```python
from build123d import *

# Parameters (mm, degrees)
SKETCH1_R           = 31.5
SKETCH1_R_2         = 26
BOSS_EXTRUDE1_DEPTH = 35
SKETCH1_9_W         = 20
SKETCH1_9_H         = 6
SKETCH1_9_R         = 12
BOSS_EXTRUDE2_DEPTH = 21
BOSS_EXTRUDE4_START = -21
SKETCH1_13_W        = 20
SKETCH1_13_H        = 6
BOSS_EXTRUDE4_DEPTH = 42
FILLET1_R           = 72
CUT_EXTRUDE1_START  = -2.5
SKETCH1_10_W        = 150
SKETCH1_10_H        = 6
CUT_EXTRUDE1_DEPTH  = 270.112775841
SKETCH1_11_R        = 5
BOSS_EXTRUDE3_DEPTH = 21
SKETCH1_12_R        = 5
CUT_EXTRUDE2_DEPTH  = 14


with BuildPart() as part:
    # Sketch1 → Boss-Extrude1 (new, symmetric)
    with BuildSketch(Plane.XY):
        Circle(SKETCH1_R)
        Circle(SKETCH1_R_2, mode=Mode.SUBTRACT)
    extrude(amount=BOSS_EXTRUDE1_DEPTH, both=True)

    # Sketch1<9> → Boss-Extrude2 (add, symmetric)
    with BuildSketch(Plane.XY):
        with BuildLine():
            ThreePointArc((240.444891614, 14.661169931), (230.786453061, 10.283897205), (220.260411081, 9))
            Line((220.260411081, 9), (90, 13))
            Line((90, 13), (28.692333471, 13))
            ThreePointArc((28.692333471, 13), (31.5, 0), (28.692333471, -13))
            Line((28.692333471, -13), (90, -13))
            Line((90, -13), (220.260411081, -9))
            ThreePointArc((220.260411081, -9), (230.786453061, -10.283897205), (240.444891614, -14.661169931))
            ThreePointArc((240.444891614, -14.661169931), (267.5, 0), (240.444891614, 14.661169931))
        make_face()
        with Locations((80, 0)):
            Rectangle(SKETCH1_9_W, SKETCH1_9_H, mode=Mode.SUBTRACT)
        with Locations(Location((250, 0, 0), (0, 0, 180))):
            Circle(SKETCH1_9_R, mode=Mode.SUBTRACT)
    extrude(amount=BOSS_EXTRUDE2_DEPTH, both=True)

    # Sketch1<13> → Boss-Extrude4 (add)
    with BuildSketch(Plane.XY.offset(BOSS_EXTRUDE4_START)):
        with Locations((80, 0)):
            Rectangle(SKETCH1_13_W, SKETCH1_13_H)
    extrude(amount=BOSS_EXTRUDE4_DEPTH)

    # Fillet1
    fillet1_edges = [part.edges().sort_by_distance(p)[0] for p in [
        (28.692333471, 13, 0),
        (28.692333471, -13, 0),
    ]]
    fillet(fillet1_edges, radius=FILLET1_R)

    # Sketch1<10> → Cut-Extrude1 (cut, through all)
    with BuildSketch(Plane.XY.offset(CUT_EXTRUDE1_START)):
        with Locations((145, 0)):
            Rectangle(SKETCH1_10_W, SKETCH1_10_H)
        with BuildLine():
            ThreePointArc((220, 3), (223, 0), (220, -3))
            Line((220, -3), (220, 3))
        make_face()
        with BuildLine():
            Line((70, -3), (70, 3))
            ThreePointArc((70, 3), (67, 0), (70, -3))
        make_face()
    cut_extrude1 = extrude(amount=-CUT_EXTRUDE1_DEPTH, mode=Mode.SUBTRACT)

    # Mirror1: Cut-Extrude1 across plane
    add(cut_extrude1.mirror(Plane.XY), mode=Mode.SUBTRACT)

    # Sketch1<11> → Boss-Extrude3 (add, symmetric)
    with BuildSketch(Plane.XY):
        with BuildLine():
            Line((28.692333471, 13), (90, 13))
            ThreePointArc((90, 13), (54.465075477, 23.652725045), (28.950381961, 50.582482314))
            ThreePointArc((28.950381961, 50.582482314), (18.050555131, 58.582082925), (4.938808192, 55.283306326))
            ThreePointArc((4.938808192, 55.283306326), (-15.790013542, 43.424058768), (-39.257670087, 38.997446139))
            ThreePointArc((-39.257670087, 38.997446139), (-49.580007549, 33.5540347), (-51.376901133, 22.023529412))
            ThreePointArc((-51.376901133, 22.023529412), (-47.925892025, 0), (-51.376901133, -22.023529412))
            ThreePointArc((-51.376901133, -22.023529412), (-49.563579479, -33.576990734), (-39.201221462, -38.998442596))
            ThreePointArc((-39.201221462, -38.998442596), (-14.290092236, -43.85808942), (7.387013832, -57.059740797))
            ThreePointArc((7.387013832, -57.059740797), (18.504940725, -60.078747549), (27.655633909, -53.079639433))
            ThreePointArc((27.655633909, -53.079639433), (53.274598705, -24.401721259), (90, -13))
            Line((90, -13), (28.692333471, -13))
            ThreePointArc((28.692333471, -13), (-31.5, 0), (28.692333471, 13))
        make_face()
        with Locations(Location((16, -47.322365932, 0), (0, 0, 180))):
            Circle(SKETCH1_11_R, mode=Mode.SUBTRACT)
        with Locations(Location((-39, -26, 0), (0, 0, 180))):
            Circle(SKETCH1_11_R, mode=Mode.SUBTRACT)
        with Locations(Location((-39, 26, 0), (0, 0, 180))):
            Circle(SKETCH1_11_R, mode=Mode.SUBTRACT)
        with Locations(Location((15, 43, 0), (0, 0, 180))):
            Circle(SKETCH1_11_R, mode=Mode.SUBTRACT)
    extrude(amount=BOSS_EXTRUDE3_DEPTH, both=True)

    # Sketch1<12> → Cut-Extrude2 (cut, symmetric)
    with BuildSketch(Plane.XY):
        with BuildLine():
            Line((28.692333471, 13), (90, 13))
            ThreePointArc((90, 13), (54.465075477, 23.652725045), (28.950381961, 50.582482314))
            ThreePointArc((28.950381961, 50.582482314), (18.050555131, 58.582082925), (4.938808192, 55.283306326))
            ThreePointArc((4.938808192, 55.283306326), (-15.790013542, 43.424058768), (-39.257670087, 38.997446139))
            ThreePointArc((-39.257670087, 38.997446139), (-49.580007549, 33.5540347), (-51.376901133, 22.023529412))
            ThreePointArc((-51.376901133, 22.023529412), (-47.925892025, 0), (-51.376901133, -22.023529412))
            ThreePointArc((-51.376901133, -22.023529412), (-49.563579479, -33.576990734), (-39.201221462, -38.998442596))
            ThreePointArc((-39.201221462, -38.998442596), (-14.290092236, -43.85808942), (7.387013832, -57.059740797))
            ThreePointArc((7.387013832, -57.059740797), (18.504940725, -60.078747549), (27.655633909, -53.079639433))
            ThreePointArc((27.655633909, -53.079639433), (53.274598705, -24.401721259), (90, -13))
            Line((90, -13), (28.692333471, -13))
            ThreePointArc((28.692333471, -13), (-31.5, 0), (28.692333471, 13))
        make_face()
        with Locations(Location((16, -47.322365932, 0), (0, 0, 180))):
            Circle(SKETCH1_12_R, mode=Mode.SUBTRACT)
        with Locations(Location((-39, -26, 0), (0, 0, 180))):
            Circle(SKETCH1_12_R, mode=Mode.SUBTRACT)
        with Locations(Location((-39, 26, 0), (0, 0, 180))):
            Circle(SKETCH1_12_R, mode=Mode.SUBTRACT)
        with Locations(Location((15, 43, 0), (0, 0, 180))):
            Circle(SKETCH1_12_R, mode=Mode.SUBTRACT)
    extrude(amount=CUT_EXTRUDE2_DEPTH, both=True, mode=Mode.SUBTRACT)


solid = part.part
```
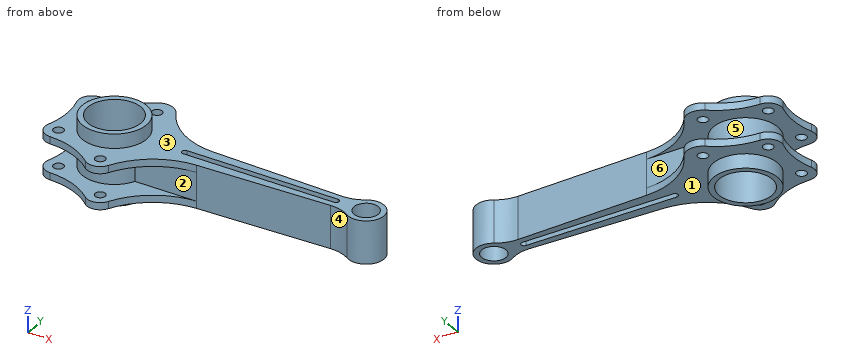
Verification items for the finished model (mm, model axes). Face numbers are marked on the shaded views. A direction names the side the tool comes from. Coordinates: 2 decimals unless noted, no trailing zeros. Order: outer loops, then holes, each group sorted by start corner. A loop starts at its lowest first (then second) coordinate and runs counter-clockwise, first axis right, second up. Notation, with made-up numbers: (64, 15.5) - (103, 15.5) arc R25 ccw to (103, 42.5) - close; hole circle Ø5 at (68.25, 10). An arc over 180 degrees is marked (long way). Return JSON: item names as keys, results as strings.
(1) Thickness scan on line 1 along Y through (x, z) = (-39, -16.25); line 2 along Z through (x, y) = (31, -21); line 3 along Y through (x, z) = (250, 4.5). Record the ranges inside material, lowest first.
Filled sheet:
{"line 1": "y = -39 to -31, -21 to 21, 31 to 39", "line 2": "z = -21 to -14, 14 to 21", "line 3": "y = -17.5 to -12, 12 to 17.5"}
(2) Section check C-C, the plane x = -8. Record the cut outline in (y, z).
Filled sheet:
{"outline": "(-46.65, -21) - (-30.47, -21) - (-30.47, -35) - (-24.74, -35) - (-24.74, 35) - (-30.47, 35) - (-30.47, 21) - (-46.65, 21) - (-46.65, 14) - (-30.47, 14) - (-30.47, -14) - (-46.65, -14) - close; (24.74, -35) - (30.47, -35) - (30.47, -21) - (46.83, -21) - (46.83, -14) - (30.47, -14) - (30.47, 14) - (46.83, 14) - (46.83, 21) - (30.47, 21) - (30.47, 35) - (24.74, 35) - close"}
(3) Access from +Z, -Z, +X, -X, +Y, -Y to the whole of each face (thin tool, end or side, straight path). Record for the marked faces 3, 4, 5 and 6.
Filled sheet:
{"face 3": "+Z", "face 4": "+Z, -Z, -Y", "face 5": "none", "face 6": "+Y"}
(4) Section check B-B, the plane z = -8. Record the cut outline in (x, y), and give its area (3 significant figures).
Filled sheet:
{"outline": "(28.69, -13) - (90, -13) - (220.26, -9) arc R35 cw to (240.44, -14.66) arc R17.5 ccw (long way) to (240.44, 14.66) arc R35 cw to (220.26, 9) - (90, 13) - (28.69, 13) arc R31.5 ccw (long way) to start; hole circle Ø52 at (0, 0); hole (70, -3) - (220, -3) arc R3 ccw to (220, 3) - (70, 3) arc R3 ccw to start; hole circle Ø24 at (250, 0)", "area": "5,250 mm^2"}
(5) Section check D-D, the plane x = 212.5. Record the cut outline in (y, z).
Filled sheet:
{"outline": "(-9.24, -21) - (-3, -21) - (-3, -2.5) - (3, -2.5) - (3, -21) - (9.24, -21) - (9.24, 21) - (3, 21) - (3, 2.5) - (-3, 2.5) - (-3, 21) - (-9.24, 21) - close"}
(6) Mould release check, pull along X, two halves, no side actions. Record for the marked faces 1 and 2: pulls with the +X half, pulls with the -X half, needs draft (parallel to the pull), parting line crosses it, or undercut.
Filled sheet:
{"face 1": "needs draft", "face 2": "undercut"}
(7) Section check A-A, the plane y = 0. Give the number of separate pieces and of enclosed holes in the cut face, and give its area (3 significant figures).
Filled sheet:
{"separate pieces": "3", "enclosed holes": "0", "area": "4,130 mm^2"}
(8) Go/stop test with flat-tipped pins: pin 1 (9 mm diameter, centred on x = 117, z = -9, fed in from -Y); pin 2 (8 mm diameter, centred on x = 207.5, y = -2, fed in from -Z); pin 3 (22.5 mm diameter, centred on x = 54, z = -6.5, fed in from -Y). Record where each tip stops, or that it passes through.
Filled sheet:
{"pin 1": "stops at y = -12.31", "pin 2": "stops at z = -21", "pin 3": "stops at y = -30.08"}
